Check sheet for the modelled part. Datum: model origin and axes. Units: mm. A direction names the side the tool comes from. Give positions to 0.01 mm unless a question says otherwise; leave off trailing zeros. Loops run counter-clockwise (first coordinate to the right, second up) from the corner with the lowest first, then second, coordinate; pieces in that order, holes last. Notation, with made-up numbers: M 23.25,5 L 29.25,5 A33 cw 29.25,35 Z; hole C 82,60.5 d8. An arc over 180 degrees is marked long. Put each result on its own line as item: value. Start each with the question number.
```python
from build123d import *

# Parameters (mm, degrees)
F0_W     = 7.95
F0_H     = 4
F1_DEPTH = 10
F2_R     = 2.6
F3_DEPTH = 21
F4_R     = 2.6
F5_DEPTH = 50
F6_R     = 3


with BuildPart() as f1:
    # F0 (on Top) → F1 (new body)
    with BuildSketch(Plane.XY):
        with BuildLine():
            Line((23.658212, 10.958917), (23.658212, 15.958917))
            Line((23.658212, 15.958917), (11.205489, 15.958917))
            Line((11.205489, 15.958917), (11.205489, 32.5))
            Line((11.205489, 32.5), (4.305489, 32.5))
            Line((4.305489, 32.5), (4.305489, 20.5))
            Line((4.305489, 20.5), (-2.894511, 20.5))
            Line((-2.894511, 20.5), (-2.894511, 32.5))
            Line((-2.894511, 32.5), (-9.794511, 32.5))
            Line((-9.794511, 32.5), (-9.794511, 16.861718))
            ThreePointArc((-9.794511, 16.861718), (-17.643481, -8.304071), (6.751771, -18.293813))
            Line((6.751771, -18.293813), (12.970301, -18.293813))
            Line((12.970301, -18.293813), (23.658212, -18.293813))
            Line((23.658212, -18.293813), (23.658212, -10.293813))
            Line((23.658212, -10.293813), (11.588245, -10.293813))
            ThreePointArc((11.588245, -10.293813), (-15.493262, -0.456975), (10.961393, 10.958917))
            Line((10.961393, 10.958917), (23.658212, 10.958917))
        make_face()
        with Locations((17.683212, -14.293813)):
            Rectangle(F0_W, F0_H, mode=Mode.SUBTRACT)
    extrude(amount=F1_DEPTH)

    # F2 (on face) → F3 (cut, through all)
    with BuildSketch(Plane.YZ.offset(11.205489)):
        with BuildLine():
            ThreePointArc((32.5, 5), (31.035534, 1.464466), (27.5, 0))
            Line((27.5, 0), (32.5, 0))
            Line((32.5, 0), (32.5, 5))
        make_face()
        with BuildLine():
            ThreePointArc((27.5, 10), (31.035534, 8.535534), (32.5, 5))
            Line((32.5, 5), (32.5, 10))
            Line((32.5, 10), (27.5, 10))
        make_face()
        with Locations((27.5, 5)):
            Circle(F2_R)
    extrude(amount=-F3_DEPTH, mode=Mode.SUBTRACT)

    # F4 (on face) → F5 (cut, symmetric)
    with BuildSketch(Plane(origin=(0, -16.293813, 0), x_dir=(-1, 0, 0), z_dir=(0, 1, 0))):
        with Locations((-17.683212, 5)):
            Circle(F4_R)
    extrude(amount=F5_DEPTH, both=True, mode=Mode.SUBTRACT)

    # F6
    f6_edges = [f1.edges().sort_by_distance(p)[0] for p in [
        (23.658212, 15.958917, 5),
        (23.658212, -10.293813, 5),
        (23.658212, -18.293813, 5),
    ]]
    fillet(f6_edges, radius=F6_R)


solid = f1.part
```
Q1. Section check B-B, the plane x = 0. Record the cut outline in (y, z).
Q2. Thickness scan on line 1 along X through (y, z) = (25, 1.5); line 2 along Y through (x, z) = (14.5, 9.5); line 3 along Y through (x, z) = (-7.5, 5.5). Record the ranges inside material, lowest first. Write a range as [from, to].
Q3. Mould release check, pull along Z, two halves, no side actions. Record for faces 1 (the face through (0, 16, 0)), 2 (the face through (-6.3, 24.9, 5.1)), 3 (the face through (15.203, 13.494, 5.781)), 4 (the face through (-9.795, 23, 5)): pulls with the +Z half, pulls with the -Z half, needs draft (parallel to the pull), parting line crosses it, or undercut.
Q4. Section check A-A, the plane y = 22. Record the cut outline in (x, z), then the cut area to 3 significant figures.
Q5. Section check D-D, the plane z = 1.75. Record the cut outline in (x, y), then the cut area to 3 significant figures.
Q6. Section check C-C, the plane x = 8. Record the cut outline in (y, z), then the cut area to 3 significant figures.
Q7. Depth check by flat-ended pin: P1, Ø4, axis at x = 19, z = 7, coming from the +Y side; P2, Ø3, axis at x = 17, z = 7, coming from the -Y side; P3, Ø3, axis at y = 17.5, z = 7, coming from the +X side. Enter the tip coordinate at first touch or a pass-through.
Q8. Access from +Z, -Z, +X, -X, +Y, -Y to the whole of each face (thin tool, end or side, straight path). Record for faces 5 (the face through (15, -10.294, 4)), 6 (the face through (1, 20.5, 5)), 7 (the face through (21.658, -14, 5)).
Found:
1. outline: M -19.5,0 L -15.5,0 L -15.5,10 L -19.5,10 Z; M 15.5,0 L 20.5,0 L 20.5,10 L 15.5,10 Z
2. line 1: x = [-9.79, -2.89], [4.31, 11.21]
2. line 2: y = [-18.29, -16.29], [-12.29, -10.29], [10.96, 15.96]
2. line 3: y = [-18, -13.56], [13.56, 24.95], [30.05, 32.47]
3. face 1: pulls with the -Z half
3. face 2: undercut
3. face 3: undercut
3. face 4: needs draft
4. outline: M -9.79,0 L -2.89,0 L -2.89,10 L -9.79,10 Z; M 4.31,0 L 11.21,0 L 11.21,10 L 4.31,10 Z
4. area: 138 mm^2
5. outline: M -9.79,16.86 A19.5 ccw 6.75,-18.29 L 20.66,-18.29 A3 ccw 23.66,-15.29 L 23.66,-13.29 A3 ccw 20.66,-10.29 L 11.59,-10.29 A15.5 cw long 10.96,10.96 L 23.66,10.96 L 23.66,12.96 A3 ccw 20.66,15.96 L 11.21,15.96 L 11.21,31.3 L 4.31,31.3 L 4.31,20.5 L -2.89,20.5 L -2.89,31.3 L -9.79,31.3 Z; hole M 13.71,-16.29 L 21.66,-16.29 L 21.66,-12.29 L 13.71,-12.29 Z
5. area: 637 mm^2
6. outline: M -18.29,0 L -13.28,0 L -13.28,10 L -18.29,10 Z; M 13.28,0 L 27.5,0 A5 ccw 27.5,10 L 13.28,10 Z; hole C 27.5,5 d5.2
6. area: 210 mm^2
7. P1: stops at y = 15.96
7. P2: stops at y = -18.29
7. P3: stops at x = 11.21
8. face 5: +Z, -Z, +X
8. face 6: +Z, -Z, +Y
8. face 7: +Z, -Z
